For this review, take the finished solid that the model builds, in its own axes (mm). A direction names the side the tool comes from. Coordinates: 2 decimals unless noted, no trailing zeros. Loops run counter-clockwise (first coordinate to the right, second up) from the corner with the lowest first, then second, coordinate; pieces in that order, holes last. Notation, with made-up numbers: (88.25, 83) - (96.25, 83) arc R17 ccw to (96.25, 97) - close; hole circle Ø9 at (52, 81.25). An arc over 180 degrees is marked (long way). Use one line per item in the form item = value. Start each with the question number.
1. Draft analysis for pull direction Z (two halves, no side actions). For faces 5 (the face through (-5.07, 11.14, -6.81)), 6 (the face through (14, -2.5, -10)), 7 (the face through (7, 0, 9)), state which applies: +Z half, -Z half, draft (parallel to the pull), parting line (faces both ways), or undercut.
2. For pin 1 Ø4 at (x, y) = (16.5, 0) entering from +Z; pin 2 Ø2.5 at (y, z) = (10, 6) entering from -X; pin 3 Ø0.8 at (y, z) = (0, -10) entering from -X; pin 4 Ø5 at (x, z) = (-19.5, -1) entering from -Y, all flat-tipped, find the tip position at first contact; note any pin that passes through.
3. To check wall thickness, follow probe 1 along X at (y, z) = (0, -10.3); probe 2 along Y at (x, z) = (17.5, -10.4); probe 3 along Y at (x, z) = (-29.5, 0). State the ranges of each line that lie inside material, in increasing order.
4. Add section A-A on y = 6. Give the boundary of the cut face in (x, z), and give its area (3 significant figures).
5. Add section D-D on y = 12.5. Give the boundary of the cut face in (x, z), and give its area (3 significant figures).
6. Add section C-C on y = 9. Give the boundary of the cut face in (x, z), and give its area (3 significant figures).
7. Machinability: for faces 1 (the face through (-20.07, 11.14, -6.81)), 2 (the face through (-41, 13, -6)), 3 (the face through (16, 1, -10)), 4 (the face through (3, -2.5, 10)), which of the approach directions +Z, -Z, +X, -X, +Y, -Y give a long, thin tool a straight path to every point of the face, cutting with its end or side? Answer none if there is none.
8. Add section B-B on x = -8. Give the boundary of the cut face in (y, z), and give its area (3 significant figures).
```python
from build123d import *

# Parameters (mm, degrees)
SKETCH1_W                = 2
SKETCH1_H                = 5
BOSS_EXTRUDE1_DEPTH      = 15
BOSS_EXTRUDE1_2_DEPTH    = 15
SKETCH2_W                = 1
SKETCH2_H                = 5
BOSS_EXTRUDE2_DEPTH      = 5
CUT_EXTRUDE1_DEPTH       = 30.107559156
CUT_EXTRUDE1_DEPTH_BACK  = 30.107559156
SKETCH3_R                = 1.5
SWEEP1_START             = 9
SWEEP1_DEPTH             = 6
BOSS_EXTRUDE3_DEPTH      = 12
CUT_EXTRUDE2_DEPTH       = 5
FILLET1_R                = 2
BOSS_EXTRUDE6_START      = -6
SKETCH7_W                = 6
SKETCH7_H                = 2
BOSS_EXTRUDE6_DEPTH      = 56
BOSS_EXTRUDE7_DEPTH      = 3
BOSS_EXTRUDE7_DEPTH_BACK = 9
SKETCH8_R                = 1.5
FILLET2_R                = 2.5
BOSS_EXTRUDE10_DEPTH     = 10
LPATTERN1_COUNT          = 2
LPATTERN1_PITCH          = 15


# Read off the part's stored shape, not the designer's step: Sweep1
with BuildPart() as part:
    # Sketch1 → Boss-Extrude1 (new body)
    with BuildSketch(Plane(origin=(0, 0, 0), x_dir=(0, 0, -1), z_dir=(1, 0, 0))):
        with Locations((-10, 0)):
            Rectangle(SKETCH1_W, SKETCH1_H)
    extrude(amount=BOSS_EXTRUDE1_DEPTH)



with BuildPart() as body_2:
    # Sketch1 → Boss-Extrude1 2 (new body)
    with BuildSketch(Plane(origin=(0, 0, 0), x_dir=(0, 0, -1), z_dir=(1, 0, 0))):
        with Locations((10, 0)):
            Rectangle(SKETCH1_W, SKETCH1_H)
    extrude(amount=BOSS_EXTRUDE1_2_DEPTH)


with BuildPart() as part_1:
    add(part.part)

    add(body_2.part)  # Boss-Extrude2 merges body 2
    # Sketch2 → Boss-Extrude2 (add)
    with BuildSketch(Plane(origin=(15, 0, 0), x_dir=(0, 0, -1), z_dir=(1, 0, 0))):
        with Locations((10.5, 0)):
            Rectangle(SKETCH2_W, SKETCH2_H)
        with Locations((-10.5, 0)):
            Rectangle(SKETCH2_W, SKETCH2_H)
    extrude(amount=BOSS_EXTRUDE2_DEPTH)

    # Sketch3 → Cut-Extrude1 (cut, two sides: drawn at the far end of the back side and taken through both)
    with BuildSketch(Plane.XY.offset(-10).offset(-CUT_EXTRUDE1_DEPTH_BACK)):
        with Locations((17.5, 0)):
            Circle(SKETCH3_R)
    extrude(amount=CUT_EXTRUDE1_DEPTH + CUT_EXTRUDE1_DEPTH_BACK, mode=Mode.SUBTRACT)

    # Sweep1 outline → Sweep1 (add)
    with BuildSketch(Plane.YZ.offset(SWEEP1_START)):
        with BuildLine():
            ThreePointArc((2.5, -11), (13.5, 0), (2.5, 11))
            Line((2.5, 11), (2.5, 9))
            ThreePointArc((2.5, 9), (11.5, 0), (2.5, -9))
            Line((2.5, -9), (2.5, -11))
        make_face()
    extrude(amount=SWEEP1_DEPTH)

    # Sketch5 → Boss-Extrude3 (add)
    with BuildSketch(Plane(origin=(0, 0, 0), x_dir=(0, 0, -1), z_dir=(1, 0, 0))):
        with BuildLine():
            Line((-9, -2.5), (-11, -2.5))
            add(Edge.make_bspline(
                [(-11, -2.5), (-11, -8.980170496), (0, -8.980170496)],
                knots=[3.141592654, 3.141592654, 3.141592654, 4.71238898, 4.71238898, 4.71238898], degree=2, weights=[1, 0.707106781, 1]))
            Line((0, -8.980170496), (0, -7.009343108))
            add(Edge.make_bspline(
                [(-9, -2.5), (-9, -7.009343108), (0, -7.009343108)],
                knots=[3.141592654, 3.141592654, 3.141592654, 4.71238898, 4.71238898, 4.71238898], degree=2, weights=[1, 0.707106781, 1]))
        make_face()
    boss_extrude3 = extrude(amount=BOSS_EXTRUDE3_DEPTH)

    # Sketch6 → Cut-Extrude2 (cut)
    with BuildSketch(Plane.ZY):
        with BuildLine():
            Line((11, -2.5), (9, -2.5))
            add(Edge.make_bspline(
                [(0, -7.009343108), (9, -7.009343108), (9, -2.5)],
                knots=[4.71238898, 4.71238898, 4.71238898, 6.283185307, 6.283185307, 6.283185307], degree=2, weights=[1, 0.707106781, 1]))
            Line((0, -7.009343108), (0, -8.980170496))
            add(Edge.make_bspline(
                [(0, -8.980170496), (11, -8.980170496), (11, -2.5)],
                knots=[4.71238898, 4.71238898, 4.71238898, 6.283185307, 6.283185307, 6.283185307], degree=2, weights=[1, 0.707106781, 1]))
        make_face()
    cut_extrude2 = extrude(amount=-CUT_EXTRUDE2_DEPTH, mode=Mode.SUBTRACT)

    # Mirror2: Boss-Extrude3, Cut-Extrude2 across plane
    add(boss_extrude3.mirror(Plane(origin=(12, -8.980170496, 0), x_dir=(1, 0, 0), z_dir=(0, 0, 1))))
    add(cut_extrude2.mirror(Plane(origin=(12, -8.980170496, 0), x_dir=(1, 0, 0), z_dir=(0, 0, 1))), mode=Mode.SUBTRACT)

    # Fillet1
    fillet1_edges = [part_1.edges().sort_by_distance(p)[0] for p in [
        (0, -2.5, -10),
        (0, 2.5, -10),
        (0, 2.5, 10),
        (0, -2.5, 10),
    ]]
    fillet(fillet1_edges, radius=FILLET1_R)

    # Sketch7 → Boss-Extrude6 (add)
    with BuildSketch(Plane.ZY.offset(-9).offset(BOSS_EXTRUDE6_START)):
        with Locations((0, 12.5)):
            Rectangle(SKETCH7_W, SKETCH7_H)
    extrude(amount=BOSS_EXTRUDE6_DEPTH)

    # Sketch8 → Boss-Extrude7 (add, two sides: drawn at the far end of the back side and taken through both)
    with BuildSketch(Plane.XY.offset(3).offset(-BOSS_EXTRUDE7_DEPTH_BACK)):
        with Locations((-41, 12.5)):
            Circle(SKETCH8_R)
    extrude(amount=BOSS_EXTRUDE7_DEPTH + BOSS_EXTRUDE7_DEPTH_BACK)

    # Fillet2
    fillet2_edges = [part_1.edges().sort_by_distance(p)[0] for p in [
        (20, -2.5, -10.5),
        (20, -2.5, 10.5),
    ]]
    fillet(fillet2_edges, radius=FILLET2_R)

    # 3DSketch3 → Boss-Extrude10 (add)
    with BuildSketch(Plane(origin=(-10, 7.995255445, 9.529017137), x_dir=(0, 0, -1), z_dir=(1, 0, 0))):
        with BuildLine():
            Line((0, 0), (2, 0))
            ThreePointArc((2, 0), (9.529017137, 3.825899604), (17.058034273, 0))
            Line((17.058034273, 0), (19.058034273, 0))
            ThreePointArc((19.058034273, 0), (15.031388903, 4.029654263), (9.529017137, 5.504744555))
            ThreePointArc((9.529017137, 5.504744555), (4.026645371, 4.029654263), (0, 0))
        make_face()
    boss_extrude10 = extrude(amount=BOSS_EXTRUDE10_DEPTH)

    # LPattern1: Boss-Extrude10 ×2
    with Locations(*[(-i * LPATTERN1_PITCH, 0, 0) for i in range(1, LPATTERN1_COUNT)]):
        add(boss_extrude10)


solid = part_1.part
```
Conclusion:
q1.face_5 = -Z half
q1.face_6 = draft
q1.face_7 = undercut
q2.pin_1 = 11
q2.pin_2 = -41.83
q2.pin_3 = 0
q2.pin_4 = 11.14
q3.probe_1 = 0 to 16, 19 to 20
q3.probe_2 = -2.5 to -1.5, 1.5 to 2.5
q3.probe_3 = 11.5 to 13.5
q4.outline = (9, -10.43) - (15, -10.43) - (15, -8.29) - (9, -8.29) - close; (9, 8.29) - (15, 8.29) - (15, 10.43) - (9, 10.43) - close
q4.area = 25.6 mm^2
q5.outline = (-42.5, -6) - (-39.5, -6) - (-39.5, -3) - (-25, -3) - (-25, -4.58) - (-15, -4.58) - (-15, -3) - (-10, -3) - (-10, -4.58) - (0, -4.58) - (0, -3) - (9, -3) - (9, -4.58) - (15, -4.58) - (15, 4.58) - (9, 4.58) - (9, 3) - (0, 3) - (0, 4.58) - (-10, 4.58) - (-10, 3) - (-15, 3) - (-15, 4.58) - (-25, 4.58) - (-25, 3) - (-39.5, 3) - (-39.5, 6) - (-42.5, 6) - close
q5.area = 445 mm^2
q6.outline = (-25, -8.87) - (-15, -8.87) - (-15, -6.68) - (-25, -6.68) - close; (-25, 6.68) - (-15, 6.68) - (-15, 8.87) - (-25, 8.87) - close; (-10, -8.87) - (0, -8.87) - (0, -6.68) - (-10, -6.68) - close; (-10, 6.68) - (0, 6.68) - (0, 8.87) - (-10, 8.87) - close; (9, -8.87) - (15, -8.87) - (15, -6.22) - (9, -6.22) - close; (9, 6.22) - (15, 6.22) - (15, 8.87) - (9, 8.87) - close
q6.area = 120 mm^2
q7.face_1 = -Z, +X, +Y
q7.face_2 = -Z, -X, +Y, -Y
q7.face_3 = +X, +Y, -Y
q7.face_4 = +Z, -Z, -X, -Y
q8.outline = (8, -9.53) arc R11 ccw to (13.08, -3) - (13.5, -3) - (13.5, 3) - (13.08, 3) arc R11 ccw to (8, 9.53) - (8, 7.53) arc R9.32 cw to (11.5, 2.43) - (11.5, -2.43) arc R9.32 cw to (8, -7.53) - close
q8.area = 36.0 mm^2
